Autodesk Inventor part; units mm, degrees
ref_plane "YZ Plane" through (0, 0, 0) normal (1, 0, 0) x (0, 1, 0)
ref_plane "XZ Plane" through (0, 0, 0) normal (0, 1, 0) x (-1, 0, 0)
ref_plane "XY Plane" through (0, 0, 0) normal (0, 0, 1) x (1, 0, 0)
sketch "Sketch1" plane through (0, 0, 0) normal (0, 0, 1) x (1, 0, 0)
  circle A0 centre (-6.35, 0) radius 1.905
  circle A1 centre (6.35, 0) radius 1.87325
  arc A2 (-6.35, 2.54) -> (-6.35, -2.54) centre (-6.35, 0) ccw
  line L0 (-6.35, 2.54) -> (4.7625, 2.54)
  line L1 (0, 3.556) -> (0, -3.556) construction
  line L2 (-12.446, 0) -> (12.446, 0) construction
  line L3 (-6.35, -2.54) -> (4.7625, -2.54)
  arc A3 (-3.453414, -2.54) -> (-3.453414, 2.54) centre (-4.7625, 0) ccw
  arc A4 (6.35, -2.54) -> (6.35, 2.54) centre (6.35, 0) ccw
  line L4 (4.7625, 2.54) -> (6.35, 2.54)
  line L5 (4.7625, -2.54) -> (6.35, -2.54)
  arc A5 (4.7625, 2.54) -> (4.7625, -2.54) centre (4.7625, 0) ccw
  dimension "d2" = 3.81
  dimension "d3" = 3.7465
  dimension "d5" = 5.08
  dimension "d6" = 12.7
  dimension "d16" = 1.5875
  dimension "d17" = 2.8575
  dimension "d18" = 1.5875
sketch "Sketch1 outline for Extrusion1" plane through (0, 0, 0) normal (0, 0, 1) x (1, 0, 0)
  arc A0 (4.7625, -2.54) -> (4.7625, 2.54) centre (4.7625, 0) cw
  line L0 (4.7625, 2.54) -> (-6.35, 2.54)
  arc A1 (-6.35, 2.54) -> (-6.35, -2.54) centre (-6.35, 0) ccw
  line L1 (-6.35, -2.54) -> (4.7625, -2.54)
  circle A2 centre (-6.35, 0) radius 1.905
extrude "Extrusion1" add sketch "Sketch1 outline for Extrusion1" along normal mid plane 25.4
sketch "Sketch1 outline for Extrusion2" plane through (0, 0, 0) normal (0, 0, 1) x (1, 0, 0)
  arc A0 (4.7625, 2.54) -> (4.7625, -2.54) centre (4.7625, 0) ccw
  line L0 (6.35, 2.54) -> (4.7625, 2.54)
  line L1 (4.7625, -2.54) -> (6.35, -2.54)
  arc A1 (6.35, -2.54) -> (6.35, 2.54) centre (6.35, 0) ccw
  circle A2 centre (6.35, 0) radius 1.87325
extrude "Extrusion2" add sketch "Sketch1 outline for Extrusion2" along normal mid plane 19.05
sketch "Sketch1 outline for Extrusion3" plane through (0, 0, 0) normal (0, 0, 1) x (1, 0, 0)
  line L0 (-3.453414, 2.54) -> (-6.35, 2.54)
  arc A0 (-3.453414, -2.54) -> (-3.453414, 2.54) centre (-4.7625, 0) ccw
  arc A1 (-6.35, 2.54) -> (-6.35, -2.54) centre (-6.35, 0) ccw
  line L1 (-6.35, -2.54) -> (-3.453414, -2.54)
  circle A2 centre (-6.35, 0) radius 1.905
extrude "Extrusion3" cut sketch "Sketch1 outline for Extrusion3" along normal mid plane 19.685
sketch "Sketch1 outline for Extrusion4" plane through (0, 0, 0) normal (0, 0, 1) x (1, 0, 0)
  circle A0 centre (6.35, 0) radius 1.87325
extrude "Extrusion4" add sketch "Sketch1 outline for Extrusion4" along normal mid plane 23.8125
chamfer "Chamfer1" distance 0.635 angle 45 2 edges at (4.4768, 0, 11.9062) (4.4768, 0, -11.9062)
fillet "Fillet1" radius 0.3175 6 edges at (-3.4534, 2.54, 0) (-3.4534, -2.54, 0) (4.7625, 2.54, 11.1125) (4.7625, 2.54, -11.1125) (4.7625, -2.54, 11.1125) (4.7625, -2.54, -11.1125)
equation "\"d18\" = d16"
properties part number "TrackDisplayStrapSegment"
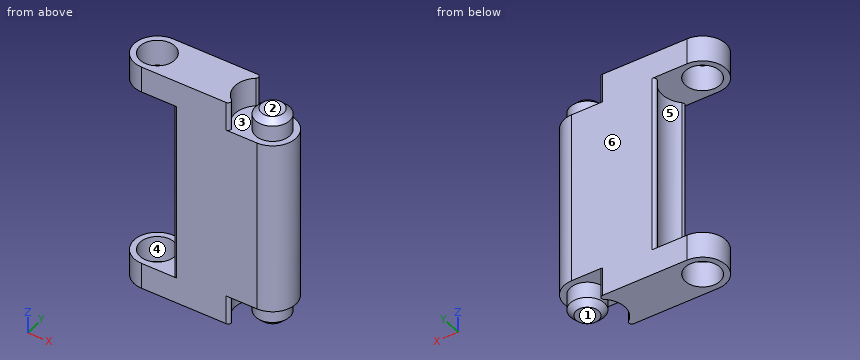
The model under review builds one solid part; all positions refer to its coordinate system, in mm. Face numbers are marked on the shaded views. A direction names the side the tool comes from. Round coordinates to 2 decimals unless told otherwise and drop trailing zeros. Order: outer loops, then holes, each group sorted by start corner. A loop starts at its lowest first (then second) coordinate and runs counter-clockwise, first axis right, second up. Notation, with made-up numbers: (46.25, 81.5) -> (102.25, 81.5) arc R8 ccw to (102.25, 85.5) -> close; hole circle Ø5 at (53, 47.25). An arc over 180 degrees is marked (long way). Use CSV: the item, a comma, the result in double quotes. Start each with the question number.
(1) Consider section A-A on y = 0. State how many separate pieces and enclosed holes the cut face has, and give its area (3 significant figures).
(2) Tool access review of the marked faces 1, 2 and 3: name each direction out of +Z, -Z, +X, -X, +Y, -Y from which nothing blocks a thin tool from reaching the whole face with its end or side.
(3) Insertion check: pin 1 (1.5 mm diameter, centred on x = 5.5, y = 0, fed in from +Z); pin 2 (2 mm diameter, centred on x = 7, y = 0.5, fed in from -Z). Each pin has a flat end and moves straight along its axis. Give the tip position at first contact, or say it passes through.
(4) Wall thickness on probe 1 along Y at (x, z) = (-6.35, -11.05) (3 decimals); probe 2 along Z at (x, y) = (7.75, -1.55) (3 decimals); probe 3 along Z at (x, y) = (-5, -1.65): over which ranges is each line inside the solid? List them lowest first. Write a range as from..to.
(5) Consider section B-B on x = -5.5. Write out the cut boundary in (y, z), and give its area (3 significant figures).
(6) Mouldability with a two-part tool opening along X and no side actions: class the marked faces 4, 5 and 6 as pulls with the +X half, pulls with the -X half, needs draft (parallel to the pull), parting line crosses it, or undercut.
Responses:
1,separate pieces,"3"
1,enclosed holes,"0"
1,area,"267 mm²"
2,face 1,"-Z, +X, +Y, -Y"
2,face 2,"+Z, +X, +Y, -Y"
2,face 3,"+Z"
3,pin 1,"z = 11.91"
3,pin 2,"z = -11.91"
4,probe 1,"-2.54..-1.905, 1.905..2.54"
4,probe 2,"-9.525..9.525"
4,probe 3,"-12.7..-9.84, 9.84..12.7"
5,outline,"(-2.54, -12.7) -> (-1.7, -12.7) -> (-1.7, -9.84) -> (-2.54, -9.84) -> close; (-2.54, 9.84) -> (-1.7, 9.84) -> (-1.7, 12.7) -> (-2.54, 12.7) -> close; (1.7, -12.7) -> (2.54, -12.7) -> (2.54, -9.84) -> (1.7, -9.84) -> close; (1.7, 9.84) -> (2.54, 9.84) -> (2.54, 12.7) -> (1.7, 12.7) -> close"
5,area,"9.55 mm²"
6,face 4,"undercut"
6,face 5,"pulls with the -X half"
6,face 6,"needs draft"
